```python
from build123d import *

# Parameters (mm, degrees)
SKETCH1_R           = 15
SKETCH1_R_2         = 10
BOSS_EXTRUDE1_DEPTH = 5
FILLET1_R           = 0.5
SKETCH2_R           = 13
SKETCH2_R_2         = 11
CUT_EXTRUDE1_DEPTH  = 0.5
SKETCH3_R           = 13
SKETCH3_R_2         = 11
CUT_EXTRUDE2_DEPTH  = 0.5


with BuildPart() as part:
    # Sketch1 → Boss-Extrude1 (new body)
    with BuildSketch(Plane.XY):
        with Locations((0, 1.584180911)):
            Circle(SKETCH1_R)
        with Locations((0, 1.584180911)):
            Circle(SKETCH1_R_2, mode=Mode.SUBTRACT)
    extrude(amount=BOSS_EXTRUDE1_DEPTH)

    # Fillet1
    fillet1_edges = [part.edges().sort_by_distance(p)[0] for p in [
        (-15, 1.584180911, 0),
        (-15, 1.584180911, 5),
    ]]
    fillet(fillet1_edges, radius=FILLET1_R)

    # Sketch2 → Cut-Extrude1 (cut)
    with BuildSketch(Plane.XY.offset(5)):
        with Locations((0, 1.584180911)):
            Circle(SKETCH2_R)
        with Locations((0, 1.584180911)):
            Circle(SKETCH2_R_2, mode=Mode.SUBTRACT)
    extrude(amount=-CUT_EXTRUDE1_DEPTH, mode=Mode.SUBTRACT)

    # Sketch3 → Cut-Extrude2 (cut)
    with BuildSketch(Plane(origin=(0, 0, 0), x_dir=(-1, 0, 0), z_dir=(0, 0, -1))):
        with Locations((0, 1.584180911)):
            Circle(SKETCH3_R)
        with Locations((0, 1.584180911)):
            Circle(SKETCH3_R_2, mode=Mode.SUBTRACT)
    extrude(amount=-CUT_EXTRUDE2_DEPTH, mode=Mode.SUBTRACT)


solid = part.part
```
Here's how the part is built. I have some questions about the finished solid (model axes, mm). A direction names the side the tool comes from. Give positions to 0.01 mm unless a question says otherwise; leave off trailing zeros. Loops run counter-clockwise (first coordinate to the right, second up) from the corner with the lowest first, then second, coordinate; pieces in that order, holes last. Notation, with made-up numbers: (9.25, 16.5) -> (55.25, 16.5) arc R17 ccw to (55.25, 27.5) -> close; hole circle Ø5 at (60, 77.5). An arc over 180 degrees is marked (long way). Use one line per item in the form item = value. Start each with the question number.
1) Thinking about a two-plate mould opening in X: for faces 1 (the face through (-2, 15, 5)), 2 (the face through (2.818, -11.107, 0.246)), 3 (the face through (-14.985, 2.244, 2.472)), 4 (the face through (-2.168, -8.178, 2.465)), which applies, +X half, -X half, draft (parallel to the pull), parting line (faces both ways), or undercut?
2) For P1, Ø2, axis at y = -4, z = 4, coming from the -X side; P2, Ø8, axis at x = 2, y = 1.5, coming from the -Z side; P3, Ø1, axis at y = 5, z = 3.5, coming from the +X side, each with a flat end and sliding along its axis, tell me the tip position at first contact or that it passes through.
3) Imagine slicing it at B-B (z = 3.75). Please give me the cut outline in (x, y).
4) Which directions (+Z, -Z, +X, -X, +Y, -Y) give clear straight access to the entire face, cutting with the end or side of a thin tool? Please do faces 5 (the face through (-2.385, -9.154, 4.754)), 6 (the face through (10, -1, 5)), 7 (the face through (11, 5, 0.5)).
5) Imagine slicing it at A-A (x = 0). Please give me the cut outline in (y, z).
6) Please list where these lines run through material, in increasing order: line 1 along Y through (x, z) = (0, 0.1); line 2 along Y through (x, z) = (0, 1.3); line 3 along Y through (x, z) = (0, 4.75).
Check values:
q1.face_1 = draft
q1.face_2 = undercut
q1.face_3 = parting line
q1.face_4 = undercut
q2.P1 = -14.28
q2.P2 = through
q2.P3 = 14.71
q3.outline = circle Ø30 at (0, 1.58); hole circle Ø20 at (0, 1.58)
q4.face_5 = +Z
q4.face_6 = +Z, +X, -X, +Y, -Y
q4.face_7 = -Z
q5.outline = (-13.42, 0.5) arc R0.5 ccw to (-12.92, 0) -> (-11.42, 0) -> (-11.42, 0.5) -> (-9.42, 0.5) -> (-9.42, 0) -> (-8.42, 0) -> (-8.42, 5) -> (-9.42, 5) -> (-9.42, 4.5) -> (-11.42, 4.5) -> (-11.42, 5) -> (-12.92, 5) arc R0.5 ccw to (-13.42, 4.5) -> close; (11.58, 0) -> (12.58, 0) -> (12.58, 0.5) -> (14.58, 0.5) -> (14.58, 0) -> (16.08, 0) arc R0.5 ccw to (16.58, 0.5) -> (16.58, 4.5) arc R0.5 ccw to (16.08, 5) -> (14.58, 5) -> (14.58, 4.5) -> (12.58, 4.5) -> (12.58, 5) -> (11.58, 5) -> close
q6.line_1 = -13.22 to -11.42, -9.42 to -8.42, 11.58 to 12.58, 14.58 to 16.38
q6.line_2 = -13.42 to -8.42, 11.58 to 16.58
q6.line_3 = -13.35 to -11.42, -9.42 to -8.42, 11.58 to 12.58, 14.58 to 16.52
